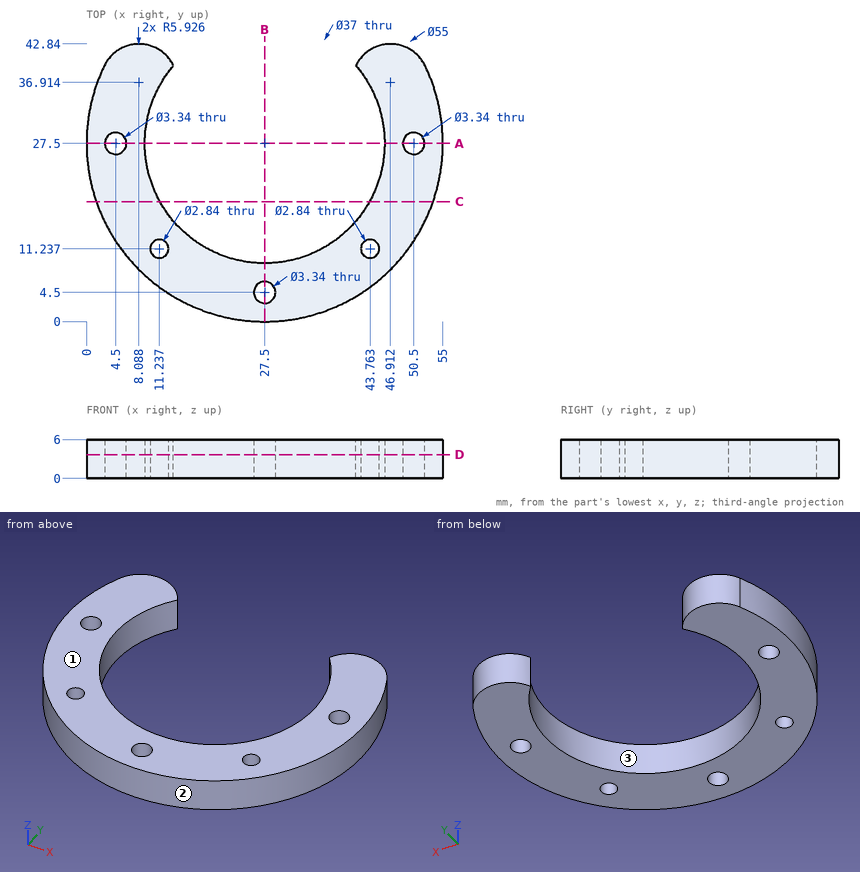
Source: three-view drawing plus pictorial views. Frame: mm from the lowest corner of the part. Give positions to 0.01 mm unless a question says otherwise; leave off trailing zeros. Order: outer loops, then holes, each group sorted by start corner. A loop starts at its lowest first (then second) coordinate and runs counter-clockwise, first axis right, second up. Notation, with made-up numbers: M -37.5,80 L -4.5,80 A19 cw -4.5,91 Z; hole C 59.25,-28.5 d1. An arc over 180 degrees is marked long. Return JSON: item names as keys, results as strings.
1) Section query D-D on z = 3.7. Output: boundary loops of the cut face in (x, y) (1 decimal).
Taken from the geometry:
{"outline": "M 2.8,39.5 A27.5 ccw long 52.2,39.5 A5.9 ccw 41.6,39.5 A18.5 cw long 13.4,39.5 A5.9 ccw Z; hole C 4.5,27.5 d3.3; hole C 11.2,11.2 d2.8; hole C 27.5,4.5 d3.3; hole C 43.8,11.2 d2.8; hole C 50.5,27.5 d3.3"}
2) Section query B-B on x = 27.5. Output: boundary loops of the cut face in (y, z).
Taken from the geometry:
{"outline": "M 0,0 L 2.83,0 L 2.83,6 L 0,6 Z; M 6.17,0 L 9,0 L 9,6 L 6.17,6 Z"}
3) Line query: L1, parallel to X at y = 11.5, z = 4.4 (1 decimal); L2, parallel to Y at x = 27.5, z = 3.15; L3, parallel to Y at x = 50.5, z = 2.8 (1 decimal). Output: solid intervals per line, ascending. Write a range as [from, to].
Taken from the geometry:
{"L1": "x = [5.1, 9.8], [12.6, 18.2], [36.8, 42.4], [45.2, 49.9]", "L2": "y = [0, 2.83], [6.17, 9]", "L3": "y = [12.4, 25.8], [29.2, 41.6]"}
4) Contact query for flat-ended pins moving along their axis: pin 1 (1.7 mm diameter, centred on x = 43.76, y = 11.24, fed in from -Z); pin 2 (1 mm diameter, centred on x = 35.5, z = 3, fed in from +Y); pin 3 (1.5 mm diameter, centred on y = 5.5, z = 1.5, fed in from -X) (1 decimal); pin 4 (1 mm diameter, centred on x = 27.5, z = 4.5, fed in from -Y). Output: stop coordinate, or through.
Taken from the geometry:
{"pin 1": "passes through", "pin 2": "stops at y = 11.07", "pin 3": "stops at x = 10", "pin 4": "stops at y = 0"}
5) Mould query, pull axis X, two halves, no side actions, for the marked faces 1, 2 and 3. Classes: released by +X, released by -X, zero draft, split by the parting line, or undercut.
Taken from the geometry:
{"face 1": "zero draft", "face 2": "split by the parting line", "face 3": "undercut"}
6) Section query A-A on y = 27.5. Output: boundary loops of the cut face in (x, z).
Taken from the geometry:
{"outline": "M 0,0 L 2.83,0 L 2.83,6 L 0,6 Z; M 6.17,0 L 9,0 L 9,6 L 6.17,6 Z; M 46,0 L 48.83,0 L 48.83,6 L 46,6 Z; M 52.17,0 L 55,0 L 55,6 L 52.17,6 Z"}
7) Section query C-C on y = 18.5. Output: boundary loops of the cut face in (x, z) (1 decimal).
Taken from the geometry:
{"outline": "M 1.5,0 L 11.3,0 L 11.3,6 L 1.5,6 Z; M 43.7,0 L 53.5,0 L 53.5,6 L 43.7,6 Z"}
